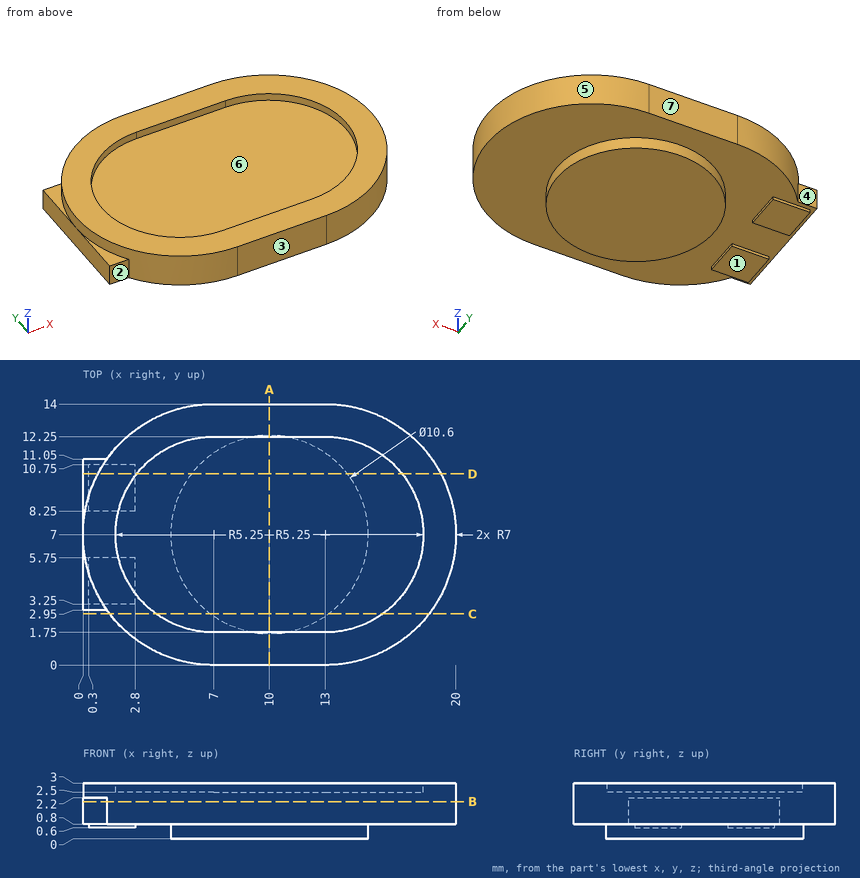
Input: dimensioned drawing with shaded views. Units: mm. Origin: part minimum x, y, z. A direction names the side the tool comes from. Round coordinates to 2 decimals unless told otherwise and drop trailing zeros. Order: outer loops, then holes, each group sorted by start corner. A loop starts at its lowest first (then second) coordinate and runs counter-clockwise, first axis right, second up.
1. Mould query, pull axis X, two halves, no side actions, for the marked faces 5, 6 and 7. Classes: released by +X, released by -X, zero draft, split by the parting line, or undercut.
The answers:
face 5: released by +X
face 6: undercut
face 7: zero draft
2. Pin query (flat end, axial travel): P1, Ø1.5, axis at x = 7, y = 8, coming from the +Z side; P2, Ø1, axis at x = 0.5, z = 1.5, coming from the +Y side; P3, Ø0.8, axis at x = 2, y = 9.5, coming from the -Z side. Return the tip coordinate at first contact, or that it passes through.
The answers:
P1: stops at z = 2.5
P2: stops at y = 11.05
P3: stops at z = 0.6
3. Cut plane B-B, the plane z = 2. Output: boundary loops of the cut face in (x, y), then the cut area to 3 significant figures.
The answers:
outline: (0, 2.95) - (1.29, 2.95) arc R7 ccw to (7, 0) - (13, 0) arc R7 ccw to (13, 14) - (7, 14) arc R7 ccw to (1.29, 11.05) - (0, 11.05) - close
area: 241 mm2
4. Cut plane D-D, the plane y = 10.25. Output: boundary loops of the cut face in (x, z).
The answers:
outline: (0, 0.8) - (0.3, 0.8) - (0.3, 0.6) - (2.8, 0.6) - (2.8, 0.8) - (5.81, 0.8) - (5.81, 0) - (14.19, 0) - (14.19, 0.8) - (19.2, 0.8) - (19.2, 3) - (17.12, 3) - (17.12, 2.5) - (2.88, 2.5) - (2.88, 3) - (0.8, 3) - (0.8, 2.2) - (0, 2.2) - close
5. Cut plane A-A, the plane x = 10. Output: boundary loops of the cut face in (y, z).
The answers:
outline: (0, 0.8) - (1.7, 0.8) - (1.7, 0) - (12.3, 0) - (12.3, 0.8) - (14, 0.8) - (14, 3) - (12.25, 3) - (12.25, 2.5) - (1.75, 2.5) - (1.75, 3) - (0, 3) - close
6. Material intervals for line 1 (Y direction, x = 9.5, z = 2.85); line 2 (Z direction, x = 7.5, y = 12.5); line 3 (X direction, y = 10.25, z = 0.65), sorted ascending.
The answers:
line 1: y = 0 to 1.75, 12.25 to 14
line 2: z = 0.8 to 3
line 3: x = 0.3 to 2.8, 5.81 to 14.19
7. Cut plane C-C, the plane y = 2.75. Output: boundary loops of the cut face in (x, z), then the cut area to 3 significant figures.
The answers:
outline: (1.44, 0.8) - (6.83, 0.8) - (6.83, 0) - (13.17, 0) - (13.17, 0.8) - (18.56, 0.8) - (18.56, 3) - (16.08, 3) - (16.08, 2.5) - (3.92, 2.5) - (3.92, 3) - (1.44, 3) - close
area: 36.7 mm2
8. Set-up query: the marked faces 1, 2, 3 and 4. Return all of +Z, -Z, +X, -X, +Y, -Y with unobstructed straight access to the full face (end or side cutting, diameter ignored); none if empty.
The answers:
face 1: -Z, -X, +Y, -Y
face 2: +Z, -Z, -X, -Y
face 3: +Z, -Z, +X, -X, -Y
face 4: +Z, -Z, -X, +Y
